For this review, take the finished solid that the model builds, in its own axes (mm). Give positions to 0.01 mm unless a question says otherwise; leave off trailing zeros. Loops run counter-clockwise (first coordinate to the right, second up) from the corner with the lowest first, then second, coordinate; pieces in that order, holes last. Notation, with made-up numbers: (3.5, -5) - (40.5, -5) arc R31 cw to (40.5, 22) - close; hole circle Ø3 at (-22, -35.5). An arc over 180 degrees is marked (long way). Answer in a Markdown table with one row per item.
```python
from build123d import *

# Parameters (mm, degrees)
BASE_FLANGE1_DEPTH             = 3.175
SKETCH11_R                     = 8
CUT_EXTRUDE1_CENTER_HOLE_DEPTH = 234.912720759
M5_CLEARANCE_HOLE1_EDGE_D      = 5.8
CUT_EXTRUDE2_DEPTH             = 234.912720759
BOSS_EXTRUDE3_DEPTH            = 3.175
M4_CLEARANCE_HOLE1_D           = 4.5
FILLET1_R                      = 2
FILLET1_OF_MIRROR1_R           = 2
FILLET2_R                      = 100


# Sheet-metal steps are written as plain solids
with BuildPart() as part:
    # Sketch1 → Base-Flange1 (new body)
    with BuildSketch(Plane(origin=(0, 0, 0), x_dir=(1, 0, 0), z_dir=(0, 1, 0))):
        with BuildLine():
            Line((226, -13.432371654), (-226, -13.432371654))
            ThreePointArc((-226, -13.432371654), (-233.502570944, -6.12369062), (-226.392788824, 1.567628346))
            Line((-226.392788824, 1.567628346), (0, 13.432371654))
            Line((0, 13.432371654), (226.392788824, 1.567628346))
            ThreePointArc((226.392788824, 1.567628346), (233.502570944, -6.12369062), (226, -13.432371654))
        make_face()
    extrude(amount=-BASE_FLANGE1_DEPTH)

    # Sketch11 → Cut-Extrude1_Center Hole (cut, through all)
    with BuildSketch(Plane(origin=(0, 0, 0), x_dir=(1, 0, 0), z_dir=(0, 1, 0))):
        with Locations(Location((0, 0, 0), (0, 0, 270))):
            Circle(SKETCH11_R)
    extrude(amount=-CUT_EXTRUDE1_CENTER_HOLE_DEPTH, mode=Mode.SUBTRACT)

    # M5 Clearance Hole1_Edge (through all)
    with Locations(Plane(origin=(0, 0, 0), x_dir=(1, 0, 0), z_dir=(0, 1, 0))):
        with Locations((-226, -5.927228885)):
            m5_clearance_hole1_edge = Hole(M5_CLEARANCE_HOLE1_EDGE_D / 2)

    # Sketch12 → Cut-Extrude2 (cut, through all)
    with BuildSketch(Plane(origin=(0, 0, 0), x_dir=(1, 0, 0), z_dir=(0, 1, 0))):
        with BuildLine():
            Line((-209.269000639, -3.543186018), (-113.515692218, 1.475032235))
            Line((-113.515692218, 1.475032235), (-113.515692218, -7.432371654))
            Line((-113.515692218, -7.432371654), (-209.167158729, -7.432371654))
            ThreePointArc((-209.167158729, -7.432371654), (-209.105791208, -5.484838459), (-209.269000639, -3.543186018))
        make_face()
        with BuildLine():
            Line((-107.515692218, 1.789478911), (-107.515692218, -7.432371654))
            Line((-107.515692218, -7.432371654), (-11.864225706, -7.432371654))
            ThreePointArc((-11.864225706, -7.432371654), (-13.994914166, -0.377329415), (-12.247479508, 6.782274375))
            Line((-12.247479508, 6.782274375), (-107.515692218, 1.789478911))
        make_face()
    cut_extrude2 = extrude(amount=-CUT_EXTRUDE2_DEPTH, mode=Mode.SUBTRACT)

    # Sketch16 → Boss-Extrude3 (add)
    with BuildSketch(Plane(origin=(0, 0, 0), x_dir=(1, 0, 0), z_dir=(0, 1, 0))):
        with BuildLine():
            Line((-113.515692218, -7.432371654), (-113.515692218, -2.978669709))
            Line((-113.515692218, -2.978669709), (-113.515692218, 1.475032235))
            Line((-113.515692218, 1.475032235), (-114.686004205, 1.413698783))
            ThreePointArc((-114.686004205, 1.413698783), (-116.513510347, -3.061853233), (-114.447375484, -7.432371654))
            Line((-114.447375484, -7.432371654), (-113.515692218, -7.432371654))
        make_face()
        with BuildLine():
            Line((-107.515692218, 1.789478911), (-107.515692218, -2.821446372))
            Line((-107.515692218, -2.821446372), (-107.515692218, -7.432371654))
            Line((-107.515692218, -7.432371654), (-106.584008951, -7.432371654))
            ThreePointArc((-106.584008951, -7.432371654), (-105.057208014, -5.391031786), (-104.515692218, -2.900058041))
            ThreePointArc((-104.515692218, -2.900058041), (-105.122208313, -0.271307126), (-106.819136008, 1.825983875))
            Line((-106.819136008, 1.825983875), (-107.515692218, 1.789478911))
        make_face()
        with BuildLine():
            ThreePointArc((-200, -5.40297223), (-200.117942339, -4.219165794), (-200.467132559, -3.081899659))
            Line((-200.467132559, -3.081899659), (-209.269000639, -3.543186018))
            ThreePointArc((-209.269000639, -3.543186018), (-209.105791208, -5.484838459), (-209.167158729, -7.432371654))
            Line((-209.167158729, -7.432371654), (-200.353626121, -7.432371654))
            ThreePointArc((-200.353626121, -7.432371654), (-200.089067617, -6.432961727), (-200, -5.40297223))
        make_face()
        with BuildLine():
            Line((-209.269000639, -3.543186018), (-200.467132559, -3.081899659))
            ThreePointArc((-200.467132559, -3.081899659), (-211.997958883, -5.559462595), (-200.353626121, -7.432371654))
            Line((-200.353626121, -7.432371654), (-209.167158729, -7.432371654))
            ThreePointArc((-209.167158729, -7.432371654), (-209.105791208, -5.484838459), (-209.269000639, -3.543186018))
        make_face()
    boss_extrude3 = extrude(amount=-BOSS_EXTRUDE3_DEPTH)

    # M4 Clearance Hole1 (through all)
    with Locations(Plane(origin=(0, 0, 0), x_dir=(1, 0, 0), z_dir=(0, 1, 0))):
        with Locations((-206, -5.40297223), (-110.515692218, -2.900058041)):
            m4_clearance_hole1 = Hole(M4_CLEARANCE_HOLE1_D / 2)

    # Fillet1
    fillet1_edges = [part.edges().sort_by_distance(p)[0] for p in [
        (-12.247479508, -1.5875, -6.782274375),
        (-11.864225706, -1.5875, 7.432371654),
        (-114.447375484, -1.5875, 7.432371654),
        (-114.686004205, -1.5875, -1.413698783),
        (-106.819136008, -1.5875, -1.825983875),
        (-106.584008951, -1.5875, 7.432371654),
        (-200.467132559, -1.5875, 3.081899659),
        (-200.353626121, -1.5875, 7.432371654),
    ]]
    fillet(fillet1_edges, radius=FILLET1_R)

    # Mirror1: M5 Clearance Hole1_Edge, Cut-Extrude2, Boss-Extrude3, M4 Clearance Hole1 across plane
    add(m5_clearance_hole1_edge.mirror(Plane(origin=(0, 0, 0), x_dir=(0, 0, 1), z_dir=(1, 0, 0))), mode=Mode.SUBTRACT)
    add(cut_extrude2.mirror(Plane(origin=(0, 0, 0), x_dir=(0, 0, 1), z_dir=(1, 0, 0))), mode=Mode.SUBTRACT)
    add(boss_extrude3.mirror(Plane(origin=(0, 0, 0), x_dir=(0, 0, 1), z_dir=(1, 0, 0))))
    add(m4_clearance_hole1.mirror(Plane(origin=(0, 0, 0), x_dir=(0, 0, 1), z_dir=(1, 0, 0))), mode=Mode.SUBTRACT)

    # Fillet1 of Mirror1
    fillet1_of_mirror1_edges = [part.edges().sort_by_distance(p)[0] for p in [
        (12.247479508, -1.5875, -6.782274375),
        (11.864225706, -1.5875, 7.432371654),
        (114.447375484, -1.5875, 7.432371654),
        (114.686004205, -1.5875, -1.413698783),
        (106.819136008, -1.5875, -1.825983875),
        (106.584008951, -1.5875, 7.432371654),
        (200.467132559, -1.5875, 3.081899659),
        (200.353626121, -1.5875, 7.432371654),
    ]]
    fillet(fillet1_of_mirror1_edges, radius=FILLET1_OF_MIRROR1_R)

    # Fillet2
    fillet2_edges = [part.edges().sort_by_distance(p)[0] for p in [
        (0, -1.5875, -13.432371654),
    ]]
    fillet(fillet2_edges, radius=FILLET2_R)


solid = part.part
```
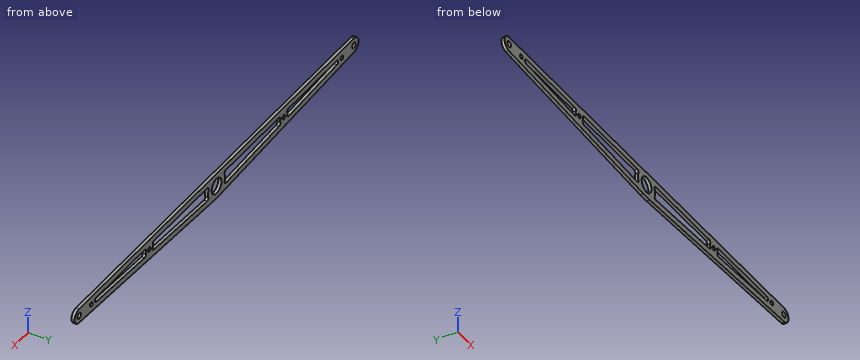
1. Clearance check with flat-ended pins moving along their axes: pin 1 (2 mm diameter, centred on x = 146.5, z = 5, fed in from -Y); pin 2 (3 mm diameter, centred on x = 126.5, z = 7, fed in from +Y); pin 3 (1.6 mm diameter, centred on x = 140, y = -2, fed in from -Z); pin 4 (1.6 mm diameter, centred on x = -45, y = -2.5, fed in from -Z). State where each tip first meets the part, or that it passes through.
Values:
| item | result |
|---|---|
| pin 1 | passes through |
| pin 2 | stops at y = 0 |
| pin 3 | stops at z = -6.14 |
| pin 4 | stops at z = -11.12 |
2. We need section C-C, the plane x = 123. Give the boundary of the cut face in (y, z) (3 decimals).
Values:
| item | result |
|---|---|
| outline | (-3.175, -6.986) - (0, -6.986) - (0, -0.978) - (-3.175, -0.978) - close; (-3.175, 7.432) - (0, 7.432) - (0, 13.432) - (-3.175, 13.432) - close |
3. We need section A-A, the plane x = 0. Give the boundary of the cut face in (y, z) (3 decimals).
Values:
| item | result |
|---|---|
| outline | (-3.175, -13.295) - (0, -13.295) - (0, -8) - (-3.175, -8) - close; (-3.175, 8) - (0, 8) - (0, 13.432) - (-3.175, 13.432) - close |
4. We need section B-B, the plane y = -1.15. Count the separate pieces of the cut face and the enclosed holes in it, and give its area (3 significant figures).
Values:
| item | result |
|---|---|
| separate pieces | 1 |
| enclosed holes | 11 |
| area | 6,090 mm^2 |
5. Wall thickness on line 1 (Z direction, x = -196, y = -0.7); line 2 (Z direction, x = -131.5, y = -1.75); line 3 (X direction, y = -0.9, z = 10): over which ranges is each line inside the solid? List them lowest first. Write a range as [from, to].
Values:
| item | result |
|---|---|
| line 1 | z = [-3.16, 2.85], [7.43, 13.43] |
| line 2 | z = [-6.54, -0.53], [7.43, 13.43] |
| line 3 | x = [-232.3, 232.3] |
